```python
from build123d import *

# Parameters (mm, degrees)
F0_R     = 2.85
F1_DEPTH = 13
F2_R     = 2
F3_DEPTH = 12.5
F4_R     = 2
F5_DEPTH = 12.5


# Not quite as in the source:
# - a feature names something its author has since deleted; it is built from what else it names


with BuildPart() as f1:
    # F0 (on Front) → F1 (new body)
    with BuildSketch(Plane.XZ):
        with BuildLine():
            ThreePointArc((3.5707142143, -3.5), (4.6289075964, -1.8902948088), (5, 0))
            ThreePointArc((5, 0), (4.6289075964, 1.8902948088), (3.5707142143, 3.5))
            Line((3.5707142143, 3.5), (-3.5707142143, 3.5))
            ThreePointArc((-3.5707142143, 3.5), (-5, 0), (-3.5707142143, -3.5))
            Line((-3.5707142143, -3.5), (3.5707142143, -3.5))
        make_face()
        Circle(F0_R, mode=Mode.SUBTRACT)
        with BuildLine():
            ThreePointArc((3.5707142143, 3.5), (4.6289075964, 1.8902948088), (5, 0))
            ThreePointArc((5, 0), (4.6289075964, -1.8902948088), (3.5707142143, -3.5))
            Line((3.5707142143, -3.5), (9, -3.5))
            Line((9, -3.5), (9, 3.5))
            Line((9, 3.5), (3.5707142143, 3.5))
        make_face()
        with BuildLine():
            Line((-3.5707142143, 3.5), (3.5707142143, 3.5))
            ThreePointArc((3.5707142143, 3.5), (0, 5), (-3.5707142143, 3.5))
        make_face()
        with BuildLine():
            ThreePointArc((-3.5707142143, -3.5), (0, -5), (3.5707142143, -3.5))
            Line((3.5707142143, -3.5), (-3.5707142143, -3.5))
        make_face()
        with BuildLine():
            ThreePointArc((-3.5707142143, -3.5), (-5, 0), (-3.5707142143, 3.5))
            Line((-3.5707142143, 3.5), (-9, 3.5))
            Line((-9, 3.5), (-9, -3.5))
            Line((-9, -3.5), (-3.5707142143, -3.5))
        make_face()
    extrude(amount=F1_DEPTH)

    # F2 (on Top) → F3 (cut, symmetric)
    with BuildSketch(Plane.XY):
        with Locations((6.3759502955, -6.5950173885)):
            Circle(F2_R)
    extrude(amount=F3_DEPTH, both=True, mode=Mode.SUBTRACT)

    # F4 (on Top) → F5 (cut, symmetric)
    with BuildSketch(Plane.XY):
        with Locations((-6.2739360146, -6.5290778875)):
            Circle(F4_R)
    extrude(amount=F5_DEPTH, both=True, mode=Mode.SUBTRACT)


solid = f1.part
```
CAD build for the part. Positions are in the model's coordinates, mm. A direction names the side the tool comes from. Round coordinates to 2 decimals unless told otherwise and drop trailing zeros. Order: outer loops, then holes, each group sorted by start corner. A loop starts at its lowest first (then second) coordinate and runs counter-clockwise, first axis right, second up.
Q1. Two-plate mould, pull along X, no slides. Class faces 1 (the cylindrical face through (-2.262, -6.409, -1.734)), 2 (the cylindrical face through (0, -6, -5)), 3 (the flat face through (-8, -5, 3.5)): pulls with the +X half, pulls with the -X half, needs draft (parallel to the pull), parting line crosses it, or undercut.
Q2. Slice it at C-C (y = -1.75). Write the cut outline in (x, z), and give its area (3 significant figures).
Q3. Wall check: L1, parallel to X at y = -7.25, z = 0.5; L2, parallel to Z at x = -3.5, y = -7; L3, parallel to Z at x = 6, y = -11. Give the ranges that are in metal, low to high.
Q4. Slice it at D-D (y = -5.75). Write the cut outline in (x, z).
Q5. Slice it at B-B (z = 2.25). Write the cut outline in (x, y).
Q6. Slice it at A-A (x = 0). Write the cut outline in (y, z), and give its area (3 significant figures).
Q7. Drop flat-ended pins along their axis: pin 1 (1 mm diameter, centred on x = -3, y = -10.5, fed in from -Z); pin 2 (6 mm diameter, centred on x = 6, y = -6.5, fed in from -Z); pin 3 (1.6 mm diameter, centred on x = -6.5, y = -5, fed in from +Z). Give the stop position or say it passes through.
Q8. Which spindle directions (+Z, -Z, +X, -X, +Y, -Y) get a long thin tool onto all of the face, cutting with end or side? Do faces 4 (the cylindrical face through (-5.2, -4.84, 0.05)), 5 (the flat face through (4.5, -5, 3.5)), 6 (the flat face through (-8, -5, -3.5)), 7 (the flat face through (4, -5, -3.5)). Say none if no direction does.
Results below:
1. face 1: undercut
1. face 2: parting line crosses it
1. face 3: needs draft
2. outline: (-9, -3.5) - (-3.57, -3.5) arc R5 ccw to (3.57, -3.5) - (9, -3.5) - (9, 3.5) - (3.57, 3.5) arc R5 ccw to (-3.57, 3.5) - (-9, 3.5) - close; hole circle Ø5.7 at (0, 0)
2. area: 115 mm2
3. L1: x = -9 to -8.14, -4.41 to -2.81, 2.81 to 4.49, 8.27 to 9
3. L2: z = -3.57 to 3.57
3. L3: z = -3.5 to 3.5
4. outline: (-9, -3.5) - (-8.12, -3.5) - (-8.12, 3.5) - (-9, 3.5) - close; (-4.43, -3.5) - (-3.57, -3.5) arc R5 ccw to (3.57, -3.5) - (4.56, -3.5) - (4.56, 3.5) - (3.57, 3.5) arc R5 ccw to (-3.57, 3.5) - (-4.43, 3.5) - close; (8.19, -3.5) - (9, -3.5) - (9, 3.5) - (8.19, 3.5) - close; hole circle Ø5.7 at (0, 0)
5. outline: (-9, -13) - (-1.75, -13) - (-1.75, 0) - (-9, 0) - close; (1.75, -13) - (9, -13) - (9, 0) - (1.75, 0) - close; hole circle Ø4 at (-6.27, -6.53); hole circle Ø4 at (6.38, -6.6)
6. outline: (-13, -5) - (0, -5) - (0, -2.85) - (-13, -2.85) - close; (-13, 2.85) - (0, 2.85) - (0, 5) - (-13, 5) - close
6. area: 55.9 mm2
7. pin 1: stops at z = -4.33
7. pin 2: stops at z = -4
7. pin 3: stops at z = 3.5
8. face 4: +Z, -Z
8. face 5: +Z, +X, +Y, -Y
8. face 6: -Z, -X, +Y, -Y
8. face 7: -Z, +X, +Y, -Y
